Work out the finished part from the listing and answer in its coordinate system (mm). Round coordinates to 2 decimals unless told otherwise and drop trailing zeros. Write each loop counter-clockwise with the first axis right and the second up, starting at its lowest first coordinate (ties: lowest second). Pieces come first, ordered by that corner, then holes. Notation, with made-up numbers: M 39,-26.5 L 58,-26.5 A32 cw 58,5.5 Z; hole C -17.5,8.5 d2. An arc over 180 degrees is marked long. Answer in a Markdown table with one row per item.
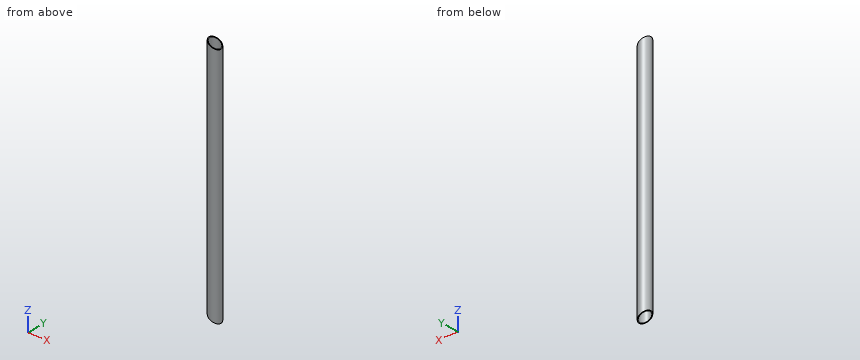
Autodesk Inventor part; units mm, degrees
ref_plane "Начальная плоскость" through (0, 0, 35.2184) normal (0, 0, 1) x (1, 0, 0)
ref_plane "Конечная плоскость" through (0, 0, 366.0401) normal (0, 0, 1) x (1, 0, 0)
ref_plane "РабПлоскость4" through (-421.1389, 19.75, 604.566) normal (0.5, 0, 0.866) x (0.866, 0, -0.5)
ref_plane "Начальная плоскость" through (0, 0, 35.2184) normal (0, 0, 1) x (1, 0, 0)
ref_plane "Конечная плоскость" through (0, 0, 366.0401) normal (0, 0, 1) x (1, 0, 0)
sketch "Эскиз" plane through (0, 0, 0) normal (0, 0, 1) x (1, 0, 0)
  circle A0 centre (0, 0) radius 7
  circle A1 centre (0, 0) radius 8
  dimension "d0" = 16
  dimension "d1" = 1
extrude "Тело" add sketch "Эскиз" along normal up to surface (330.8217 mm away) from surface at 35.2184
sketch "Sketch3" plane through (0, 0, 0) normal (0, 0, 1) x (1, 0, 0)
  line L0 (0, 0) -> (10, 0)
ref_plane "Work Plane3" through (0, 0, 0) normal (0, -1, 0) x (1, 0, 0)
sketch "Sketch4" plane through (0, 0, 0) normal (0, -1, 0) x (1, 0, 0)
  line L0 (-2, 35.2184) -> (12, 35.2184)
  line L1 (-2, 366.0401) -> (12, 366.0401)
  dimension "d7" = 330.8217
ref_plane "РабПлоскость4" through (-421.1389, 19.75, 604.566) normal (0.5, 0, 0.866) x (0.866, 0, -0.5)
split "Разделение1" plane through (-421.1389, 19.75, 604.566) removes the side toward (0.5, 0, 0.866)
ref_plane "РабПлоскость5" through (-13.9269, 193.75, 47.8779) normal (-0.5, 0, -0.866) x (-0.866, 0, 0.5)
split "Разделение2" plane through (-13.9269, 193.75, 47.8779) removes the side toward (-0.5, 0, -0.866)
equation "\"d0\" = G_H"
equation "\"d1\" = G_T"
equation "\"d2\" = G_L"
equation "\"G_H\" = 16"
equation "\"G_T\" = 1"
equation "\"G_L\" = d7"
equation "\"G_OFFSET_START\" = -35.21837"
equation "\"G_OFFSET_END\" = -72.74613"
equation "\"d4\" = -G_OFFSET_START"
equation "\"d5\" = G_OFFSET_END + B_L"
equation "\"B_L\" = 438.7862"
properties part number "Труба 16x1-330,82 ГОСТ 10704-91" material "Сталь, мягкая"
1. The part is cut by section B-B (z = 295). Determine the outline of the cut face in (x, y).
Calculated:
| item | result |
|---|---|
| outline | C 0,0 d16; hole C 0,0 d14 |
2. Consider line 1 along X through (y, z) = (-0.25, 244); line 2 along X through (y, z) = (-4.25, 178). Determine where each line is inside the solid, lowest interval first. Write a range as from..to.
Calculated:
| item | result |
|---|---|
| line 1 | x = -8..-7, 7..8 |
| line 2 | x = -6.78..-5.56, 5.56..6.78 |
3. The part is cut by section A-A (x = 0). Determine the outline of the cut face in (y, z).
Calculated:
| item | result |
|---|---|
| outline | M -8,39.84 L -7,39.84 L -7,361.42 L -8,361.42 Z; M 7,39.84 L 8,39.84 L 8,361.42 L 7,361.42 Z |
4. Given pin 1 (1.5 mm diameter, centred on x = -3.5, y = -4.5, fed in from -Z); pin 2 (4 mm diameter, centred on y = -5.5, z = 238, fed in from +X); pin 3 (1 mm diameter, centred on x = -2, z = 170.5, fed in from +Y); pin 4 (8 mm diameter, centred on y = -6, z = 286.5, fed in from -X), each flat-ended and moving along its own axis, determine where each tip first touches the part or whether it passes through.
Calculated:
| item | result |
|---|---|
| pin 1 | passes through |
| pin 2 | stops at x = 7.19 |
| pin 3 | stops at y = 7.86 |
| pin 4 | stops at x = -7.75 |
